from build123d import *

# Parameters (mm, degrees)
F0_R      = 57.15
F2_DEPTH  = 4.064
F1_R      = 39.37
F1_R_2    = 33.02
F3_DEPTH  = 11.684
F5_D      = 66.04
F7_DEPTH  = 11.685
F9_DEPTH  = 2.032
F11_DEPTH = 7.62
F13_DEPTH = 4.065


with BuildPart() as f2:
    # F0 (on Top) → F2 (new body)
    with BuildSketch(Plane.XY):
        Circle(F0_R)
    extrude(amount=F2_DEPTH)

    # F1 (on Top) → F3 (join)
    with BuildSketch(Plane.XY):
        with BuildLine():
            ThreePointArc((26.9206593113, 50.4123060596), (13.8755037511, 55.4399936477), (0, 57.15))
            ThreePointArc((0, 57.15), (-40.4111525448, -40.4111525448), (57.15, 0))
            ThreePointArc((57.15, 0), (49.013458252, 29.3905326624), (26.9206593113, 50.4123060596))
        make_face()
        with BuildLine():
            ThreePointArc((54.61, 0), (-38.6151013206, -38.6151013206), (0, 54.61))
            ThreePointArc((0, 54.61), (10.7059811808, 53.550294742), (20.9964639346, 50.4123060596))
            ThreePointArc((20.9964639346, 50.4123060596), (45.4360484388, 30.2955046544), (54.61, 0))
        make_face(mode=Mode.SUBTRACT)
        Circle(F1_R)
        Circle(F1_R_2, mode=Mode.SUBTRACT)
    extrude(amount=F3_DEPTH)

    # F5 (through all)
    with Locations(Plane(origin=(0, 0, 0), x_dir=(1, 0, 0), z_dir=(0, 0, -1))):
        with Locations((0, 0)):
            Hole(F5_D / 2)

    # F6 (on Top) → F7 (cut, through all)
    with BuildSketch(Plane.XY):
        with BuildLine():
            Line((-46.757434771, -32.8612962866), (-44.5485790293, -31.5860128296))
            ThreePointArc((-44.5485790293, -31.5860128296), (-47.2936473007, -27.305), (-49.6285790293, -22.7871947271))
            Line((-49.6285790293, -22.7871947271), (-51.837434771, -24.0624781842))
            ThreePointArc((-51.837434771, -24.0624781842), (-49.4933518263, -28.575), (-46.757434771, -32.8612962866))
        make_face()
        with BuildLine():
            Line((-28.7135911662, -20.9772086404), (-26.5001619429, -19.6992846825))
            ThreePointArc((-26.5001619429, -19.6992846825), (-28.596158833, -16.51), (-30.3101619429, -13.1001711057))
            Line((-30.3101619429, -13.1001711057), (-32.5235911662, -14.3780950636))
            ThreePointArc((-32.5235911662, -14.3780950636), (-30.7958633586, -17.78), (-28.7135911662, -20.9772086404))
        make_face()
        with BuildLine():
            Line((32.5235911662, -14.3780950636), (30.3101619429, -13.1001711057))
            ThreePointArc((30.3101619429, -13.1001711057), (28.596158833, -16.51), (26.5001619429, -19.6992846825))
            Line((26.5001619429, -19.6992846825), (28.7135911662, -20.9772086404))
            ThreePointArc((28.7135911662, -20.9772086404), (30.7958633586, -17.78), (32.5235911662, -14.3780950636))
        make_face()
        with BuildLine():
            Line((51.837434771, -24.0624781842), (49.6285790293, -22.7871947271))
            ThreePointArc((49.6285790293, -22.7871947271), (47.2936473007, -27.305), (44.5485790293, -31.5860128296))
            Line((44.5485790293, -31.5860128296), (46.757434771, -32.8612962866))
            ThreePointArc((46.757434771, -32.8612962866), (49.4933518263, -28.575), (51.837434771, -24.0624781842))
        make_face()
        with BuildLine():
            Line((-3.81, 35.355303704), (-3.81, 32.7994557882))
            ThreePointArc((-3.81, 32.7994557882), (0, 33.02), (3.81, 32.7994557882))
            Line((3.81, 32.7994557882), (3.81, 35.355303704))
            ThreePointArc((3.81, 35.355303704), (0, 35.56), (-3.81, 35.355303704))
        make_face()
        with BuildLine():
            ThreePointArc((5.08, 56.9237744708), (0, 57.15), (-5.08, 56.9237744708))
            Line((-5.08, 56.9237744708), (-5.08, 54.3732075567))
            ThreePointArc((-5.08, 54.3732075567), (0, 54.61), (5.08, 54.3732075567))
            Line((5.08, 54.3732075567), (5.08, 56.9237744708))
        make_face()
    extrude(amount=F7_DEPTH, mode=Mode.SUBTRACT)

    # F8 (on face) → F9 (cut)
    with BuildSketch(Plane(origin=(0, 0, 0), x_dir=(1, 0, 0), z_dir=(0, 0, -1))):
        with BuildLine():
            ThreePointArc((3.81, -35.355303704), (0, -35.56), (-3.81, -35.355303704))
            Line((-3.81, -35.355303704), (-3.81, -37.387303704))
            ThreePointArc((-3.81, -37.387303704), (0, -37.5809337065), (3.81, -37.387303704))
            Line((3.81, -37.387303704), (3.81, -35.355303704))
        make_face()
        with BuildLine():
            Line((-5.08, -52.3412075567), (-5.08, -54.3732075567))
            ThreePointArc((-5.08, -54.3732075567), (0, -54.61), (5.08, -54.3732075567))
            Line((5.08, -54.3732075567), (5.08, -52.3412075567))
            ThreePointArc((5.08, -52.3412075567), (0, -52.5871506025), (-5.08, -52.3412075567))
        make_face()
        with BuildLine():
            Line((32.5235911662, 14.3780950636), (34.2833547866, 15.3940950636))
            ThreePointArc((34.2833547866, 15.3940950636), (32.5460432878, 18.7904668533), (30.4733547866, 21.9932086404))
            Line((30.4733547866, 21.9932086404), (28.7135911662, 20.9772086404))
            ThreePointArc((28.7135911662, 20.9772086404), (30.7958633586, 17.78), (32.5235911662, 14.3780950636))
        make_face()
        with BuildLine():
            ThreePointArc((42.7888154088, 30.5700128296), (45.5418083344, 26.2935753012), (47.8688154088, 21.7711947271))
            Line((47.8688154088, 21.7711947271), (49.6285790293, 22.7871947271))
            ThreePointArc((49.6285790293, 22.7871947271), (47.2936473007, 27.305), (44.5485790293, 31.5860128296))
            Line((44.5485790293, 31.5860128296), (42.7888154088, 30.5700128296))
        make_face()
        with BuildLine():
            Line((-28.7135911662, 20.9772086404), (-30.4733547866, 21.9932086404))
            ThreePointArc((-30.4733547866, 21.9932086404), (-32.5460432878, 18.7904668533), (-34.2833547866, 15.3940950636))
            Line((-34.2833547866, 15.3940950636), (-32.5235911662, 14.3780950636))
            ThreePointArc((-32.5235911662, 14.3780950636), (-30.7958633586, 17.78), (-28.7135911662, 20.9772086404))
        make_face()
        with BuildLine():
            ThreePointArc((-47.8688154088, 21.7711947271), (-45.5418083344, 26.2935753012), (-42.7888154088, 30.5700128296))
            Line((-42.7888154088, 30.5700128296), (-44.5485790293, 31.5860128296))
            ThreePointArc((-44.5485790293, 31.5860128296), (-47.2936473007, 27.305), (-49.6285790293, 22.7871947271))
            Line((-49.6285790293, 22.7871947271), (-47.8688154088, 21.7711947271))
        make_face()
    extrude(amount=-F9_DEPTH, mode=Mode.SUBTRACT)

    # F10 (on face) → F11 (cut)
    with BuildSketch(Plane.XY.offset(11.684)):
        with BuildLine():
            Line((2.4859084286, -57.0959084286), (0, -54.61))
            ThreePointArc((0, -54.61), (-10.4807724417, -53.59482726), (-20.571880189, -50.5870521526))
            Line((-20.571880189, -50.5870521526), (-16.4179725703, -54.7409597713))
            ThreePointArc((-16.4179725703, -54.7409597713), (-7.0648459719, -56.7116429968), (2.4859084286, -57.0959084286))
        make_face()
    extrude(amount=-F11_DEPTH, mode=Mode.SUBTRACT)

    # F12 (on face) → F13 (cut, through all)
    with BuildSketch(Plane.XY.offset(4.064)):
        Polygon((0, 50.7088181024), (-5.08, 41.91), (5.08, 41.91), align=None)
        Polygon((-21.6871436361, 36.220467983), (-12.4055217865, 40.3529122766), (-20.6251344493, 46.3248104399), align=None)
        Polygon((-34.5443831161, 24.2680879991), (-27.7460161555, 31.8184394259), (-37.6839957789, 33.9308222046), align=None)
        Polygon((-41.4285849294, 8.1195351315), (-38.2889722665, 17.782269337), (-48.22695189, 15.6698865583), align=None)
        Polygon((-41.1494080415, -9.432959124), (-42.2114172283, 0.6713833329), (-50.4310298911, -5.3005148304), align=None)
        Polygon((-33.7551246726, -25.3544090512), (-38.8351246726, -16.5555909488), (-43.9151246726, -25.3544090512), align=None)
        Polygon((-20.5242735922, -36.8918513159), (-28.743886255, -30.9199531526), (-29.8058954418, -41.0242956095), align=None)
        Polygon((-3.7445891504, -42.0503573361), (-13.6825687739, -39.9379745574), (-10.5429561111, -49.600708763), align=None)
        Polygon((13.6825687739, -39.9379745574), (3.7445891504, -42.0503573361), (10.5429561111, -49.600708763), align=None)
        Polygon((28.743886255, -30.9199531526), (20.5242735922, -36.8918513159), (29.8058954418, -41.0242956095), align=None)
        Polygon((38.8351246726, -16.5555909488), (33.7551246726, -25.3544090512), (43.9151246726, -25.3544090512), align=None)
        Polygon((42.2114172283, 0.6713833329), (41.1494080415, -9.432959124), (50.4310298911, -5.3005148304), align=None)
        Polygon((38.2889722665, 17.782269337), (41.4285849294, 8.1195351315), (48.22695189, 15.6698865583), align=None)
        Polygon((27.7460161555, 31.8184394259), (34.5443831161, 24.2680879991), (37.6839957789, 33.9308222046), align=None)
        Polygon((12.4055217865, 40.3529122766), (21.6871436361, 36.220467983), (20.6251344493, 46.3248104399), align=None)
        Polygon((7.3743431986, -50.8387573361), (0, -42.0503573361), (-7.3743431986, -50.8387573361), align=None)
        Polygon((13.9411877648, -49.4429314341), (27.4147832292, -43.4441002391), (17.103421183, -38.4149129366), align=None)
        Polygon((32.846160712, -39.4979735122), (42.714958184, -28.5375635335), (31.2495054638, -28.1371811019), align=None)
        Polygon((46.0717340741, -22.7234571422), (50.6293288156, -8.6966228373), (39.992266357, -12.9942750364), align=None)
        Polygon((51.3310860662, -2.0198485962), (49.7894285419, 12.6480429538), (41.8200010788, 4.3954592322), align=None)
        Polygon((47.7148269492, 19.0330101218), (40.3404837506, 31.8057472143), (36.4166776913, 21.0251786681), align=None)
        Polygon((35.8482407771, 36.7948884803), (23.916302837, 45.4639488353), (24.7165798958, 34.0194537045), align=None)
        Polygon((17.7831681036, 48.1945963495), (3.3567758901, 51.2610206757), (8.7427608932, 41.1314561383), align=None)
        Polygon((-3.3567758901, 51.2610206757), (-17.7831681036, 48.1945963495), (-8.7427608932, 41.1314561383), align=None)
        Polygon((-23.916302837, 45.4639488353), (-35.8482407771, 36.7948884803), (-24.7165798958, 34.0194537045), align=None)
        Polygon((-40.3404837506, 31.8057472143), (-47.7148269492, 19.0330101218), (-36.4166776913, 21.0251786681), align=None)
        Polygon((-49.7894285419, 12.6480429538), (-51.3310860662, -2.0198485962), (-41.8200010788, 4.3954592322), align=None)
        Polygon((-50.6293288156, -8.6966228373), (-46.0717340741, -22.7234571422), (-39.992266357, -12.9942750364), align=None)
        Polygon((-42.714958184, -28.5375635335), (-32.846160712, -39.4979735122), (-31.2495054638, -28.1371811019), align=None)
        Polygon((-27.4147832292, -43.4441002391), (-13.9411877648, -49.4429314341), (-17.103421183, -38.4149129366), align=None)
    extrude(amount=-F13_DEPTH, mode=Mode.SUBTRACT)


solid = f2.part
Here's how the part is built. I have some questions about the finished solid (model axes, mm). A direction names the side the tool comes from. Coordinates: 2 decimals unless noted, no trailing zeros. Order: outer loops, then holes, each group sorted by start corner. A loop starts at its lowest first (then second) coordinate and runs counter-clockwise, first axis right, second up. Notation, with made-up numbers: M 42,67.5 L 57,67.5 A17 ccw 57,98.5 Z; hole C 89.5,10.25 d11. An arc over 180 degrees is marked long. Answer as CSV lines item,"result". Start each with the question number.
1. I want a section at A-A, the plane z = 6.5. Count the separate pieces of the cut face and the enclosed holes in it, and give its area (3 significant figures).
2. I want a section at B-B, the plane y = 3. Write out the boundary of the cut face in (x, z), and give its area (3 significant figures).
3. For pin 1 (0.7 mm diameter, centred on x = -1.5, y = 37, fed in from -Z); pin 2 (4 mm diameter, centred on y = 30.5, z = 8, fed in from -X); pin 3 (1.4 mm diameter, centred on y = 53.5, z = 8.5, fed in from +X), each with a flat end and sliding along its axis, tell me the tip position at first contact or that it passes through.
4. I want a section at C-C, the plane y = -45. Write out the boundary of the cut face in (x, z).
5. On a 3-axis mill with a long thin cutter (end or side, diameter ignored), from which of +Z, -Z, +X, -X, +Y, -Y can I reach the whole of each face in a straight line? I mean faces 1 (the cylindrical face through (-45.58, -26.23, 1)), 2 (the cylindrical face through (30.769, -17.826, 6.79)). Say none if no direction works.
6. I need wall thicknesses on line 1 (Y direction, x = 9, z = 11.25); line 2 (X direction, y = -11, z = 6); line 3 (Y direction, x = 1.5, z = 10.25). Which ranges of each line are inside material? Lowest first, please. Write a range as [from, to].
Recorded:
1,separate pieces,"5"
1,enclosed holes,"1"
1,area,"2,150 mm2"
2,outline,"M -57.07,0 L -50.8,0 L -50.8,4.06 L -54.53,4.06 L -54.53,11.68 L -57.07,11.68 Z; M -43.89,0 L -32.88,0 L -32.88,11.68 L -39.26,11.68 L -39.26,4.06 L -43.89,4.06 Z; M 32.88,0 L 43.89,0 L 43.89,4.06 L 39.26,4.06 L 39.26,11.68 L 32.88,11.68 Z; M 50.8,0 L 57.07,0 L 57.07,11.68 L 54.53,11.68 L 54.53,4.06 L 50.8,4.06 Z"
2,area,"276 mm2"
3,pin 1,"stops at z = 2.03"
3,pin 2,"stops at x = -49.54"
3,pin 3,"stops at x = 21.87"
4,outline,"M -35.23,0 L -23.92,0 L -23.92,4.06 L -30.94,4.06 L -30.94,11.68 L -35.23,11.68 Z; M -15.22,0 L -12.04,0 L -12.04,4.06 L -15.22,4.06 Z; M -6.4,0 L -2.48,0 L -2.48,4.06 L -6.4,4.06 Z; M 2.48,0 L 6.4,0 L 6.4,4.06 L 2.48,4.06 Z; M 12.04,0 L 15.22,0 L 15.22,4.06 L 12.04,4.06 Z; M 23.92,0 L 35.23,0 L 35.23,11.68 L 30.94,11.68 L 30.94,4.06 L 23.92,4.06 Z"
5,face 1,"-Z"
5,face 2,"+Z, -Z"
6,line 1,"y = [-56.44, -53.86], [-38.33, -31.77], [31.77, 38.33], [53.86, 56.44]"
6,line 2,"x = [-56.08, -53.49], [-37.8, -31.13], [31.13, 37.8], [53.49, 56.08]"
6,line 3,"y = [-56.11, -54.59], [-39.34, -32.99], [35.53, 39.34]"
